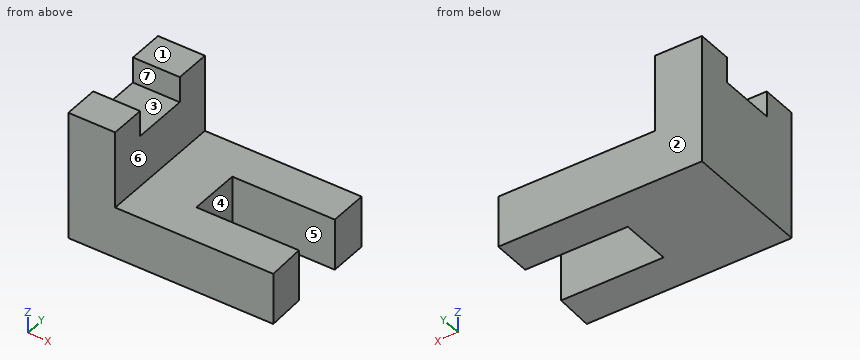
from build123d import *

# Parameters (mm, degrees)
F1_DEPTH = 50.8
F2_W     = 46.454286
F2_H     = 126.976152
F3_DEPTH = 76.2
F4_W     = 56.145773
F4_H     = 25.4
F5_DEPTH = 50.8


with BuildPart() as f1:
    # F0 (on Top) → F1 (new body)
    with BuildSketch(Plane.XY):
        Polygon((103.246617, 29.007021), (-98.60556, 29.007021), (-98.60556, -97.969131), (104.59444, -97.969131), (103.246617, -59.892979), (1.646617, -59.892979), (1.646617, -9.092979), (103.246617, -9.092979), align=None)
    extrude(amount=F1_DEPTH)

    # F2 (on face) → F3 (join)
    with BuildSketch(Plane.XY.offset(50.8)):
        with Locations((-75.378417, -34.481055)):
            Rectangle(F2_W, F2_H)
    extrude(amount=F3_DEPTH)

    # F4 (on face) → F5 (cut)
    with BuildSketch(Plane.YZ.offset(-52.151274)):
        with Locations((-34.605823, 114.3)):
            Rectangle(F4_W, F4_H)
    extrude(amount=-F5_DEPTH, mode=Mode.SUBTRACT)


solid = f1.part
CAD build for the part. Positions are in the model's coordinates, mm. Face numbers are marked on the shaded views. A direction names the side the tool comes from. Coordinates: 2 decimals unless noted, no trailing zeros. Order: outer loops, then holes, each group sorted by start corner. A loop starts at its lowest first (then second) coordinate and runs counter-clockwise, first axis right, second up.
Item 1: Band-saw the part on D-D on z = 47. List the corners of the cut face in (x, y).
Check sheet entries:
outline: (-98.61, -97.97) - (104.59, -97.97) - (103.25, -59.89) - (1.65, -59.89) - (1.65, -9.09) - (103.25, -9.09) - (103.25, 29.01) - (-98.61, 29.01) - close
Item 2: Drill centre lines: L1, parallel to X at y = -23.5, z = 29; L2, parallel to X at y = 9.5, z = 102.5; L3, parallel to Z at x = 46.5, y = 23. Where is each one in solid material? Low to high.
Check sheet entries:
L1: x = -98.61 to 1.65
L2: x = -98.61 to -52.15
L3: z = 0 to 50.8
Item 3: Two-plate mould, pull along Y, no slides. Class the marked faces 1, 2, 3 and 4: +Y half, -Y half, draft (parallel to the pull), parting line (faces both ways), or undercut.
Check sheet entries:
face 1: draft
face 2: +Y half
face 3: undercut
face 4: undercut
Item 4: Pin check, flat tips, straight feed: pin 1 Ø2 at (y, z) = (-82, 79) entering from +X; pin 2 Ø6 at (y, z) = (9, 26.5) entering from +X; pin 3 Ø12 at (y, z) = (-85, 13) entering from +X. Stop position of each tip, or through.
Check sheet entries:
pin 1: stops at x = -52.15
pin 2: stops at x = 103.25
pin 3: stops at x = 104.35
Item 5: Band-saw the part on A-A on z = 107.5. List the corners of the cut face in (x, y).
Check sheet entries:
outline: (-98.61, -97.97) - (-52.15, -97.97) - (-52.15, -62.68) - (-98.61, -62.68) - close; (-98.61, -6.53) - (-52.15, -6.53) - (-52.15, 29.01) - (-98.61, 29.01) - close
Item 6: Band-saw the part on C-C on y = -22. List the corners of the cut face in (x, z), plus the area to 3 significant figures.
Check sheet entries:
outline: (-98.61, 0) - (1.65, 0) - (1.65, 50.8) - (-52.15, 50.8) - (-52.15, 101.6) - (-98.61, 101.6) - close
area: 7,450 mm2
Item 7: 3-axis set-ups, long thin cutter, end or side, ignore diameter. For the marked faces 5, 6 and 7: which of +Z, -Z, +X, -X, +Y, -Y reach the whole face in a straight line?
Check sheet entries:
face 5: +Z, -Z, +X
face 6: +Z, +X, +Y, -Y
face 7: +Z, +X, -X
Item 8: Band-saw the part on B-B on x = -83.5. List the corners of the cut face in (y, z).
Check sheet entries:
outline: (-97.97, 0) - (29.01, 0) - (29.01, 127) - (-6.53, 127) - (-6.53, 101.6) - (-62.68, 101.6) - (-62.68, 127) - (-97.97, 127) - close
